from build123d import *

# Parameters (mm, degrees)
F1_DEPTH = 7.5
F2_R     = 5
F3_DEPTH = 10.001
F5_DEPTH = 10.001


with BuildPart() as f1:
    # F0 (on Front) → F1 (new body, symmetric)
    with BuildSketch(Plane.XZ):
        with BuildLine():
            Line((0, 10), (0, 0))
            Line((0, 0), (27.023239, 0))
            ThreePointArc((27.023239, 0), (29.876277, 0.415629), (32.492154, 1.627965))
            Line((32.492154, 1.627965), (44.251915, 9.309865))
            ThreePointArc((44.251915, 9.309865), (46.867792, 10.522202), (49.72083, 10.937831))
            Line((49.72083, 10.937831), (86.744069, 10.937831))
            Line((86.744069, 10.937831), (86.744069, 20.937831))
            Line((86.744069, 20.937831), (49.72083, 20.937831))
            ThreePointArc((49.72083, 20.937831), (46.867792, 20.522202), (44.251915, 19.309865))
            Line((44.251915, 19.309865), (32.492154, 11.627965))
            ThreePointArc((32.492154, 11.627965), (29.876277, 10.415629), (27.023239, 10))
            Line((27.023239, 10), (0, 10))
        make_face()
    extrude(amount=F1_DEPTH, both=True)

    # F2 (on face) → F3 (cut, through all)
    with BuildSketch(Plane.XY.offset(10)):
        with Locations((10, 0)):
            Circle(F2_R)
    extrude(amount=-F3_DEPTH, mode=Mode.SUBTRACT)

    # F4 (on face) → F5 (cut, through all)
    with BuildSketch(Plane.XY.offset(10)):
        with BuildLine():
            ThreePointArc((3.385622, -7.5), (0.885622, -4.114378), (0, 0))
            Line((0, 0), (0, -7.5))
            Line((0, -7.5), (3.385622, -7.5))
        make_face()
        with BuildLine():
            ThreePointArc((0, 0), (0.885622, 4.114378), (3.385622, 7.5))
            Line((3.385622, 7.5), (0, 7.5))
            Line((0, 7.5), (0, 0))
        make_face()
    extrude(amount=-F5_DEPTH, mode=Mode.SUBTRACT)


solid = f1.part
Part model, mm, in its own coordinate system. A direction names the side the tool comes from. Give positions to 0.01 mm unless a question says otherwise; leave off trailing zeros. Write each loop counter-clockwise with the first axis right and the second up, starting at its lowest first coordinate (ties: lowest second). Pieces come first, ordered by that corner, then holes.
1) Cut at A-A on x = 10. Write the cut outline in (y, z).
Resolved:
outline: (-7.5, 0) - (-5, 0) - (-5, 10) - (-7.5, 10) - close; (5, 0) - (7.5, 0) - (7.5, 10) - (5, 10) - close
2) Pin check, flat tips, straight feed: pin 1 (2 mm diameter, centred on y = -5.5, z = 15, fed in from -X); pin 2 (8 mm diameter, centred on x = 72, y = -2.5, fed in from -Z); pin 3 (5 mm diameter, centred on y = 4, z = 7, fed in from -X); pin 4 (6 mm diameter, centred on x = 10, y = 0, fed in from -Z). Stop position of each tip, or through.
Resolved:
pin 1: stops at x = 36.12
pin 2: stops at z = 10.94
pin 3: stops at x = 0.11
pin 4: passes through
3) Two-plate mould, pull along Z, no slides. Class faces 4 (the face through (86.744, 0, 16)), 5 (the face through (29.92, -0.11, 10.43)), 6 (the face through (46.8, -0.1, 10.5)): released by +Z, released by -Z, zero draft, split by the parting line, or undercut.
Resolved:
face 4: zero draft
face 5: released by +Z
face 6: released by -Z
4) Cut at D-D on y = 6. Write the cut outline in (x, z).
Resolved:
outline: (2, 0) - (27.02, 0) arc R10 ccw to (32.49, 1.63) - (44.25, 9.31) arc R10 cw to (49.72, 10.94) - (86.74, 10.94) - (86.74, 20.94) - (49.72, 20.94) arc R10 ccw to (44.25, 19.31) - (32.49, 11.63) arc R10 cw to (27.02, 10) - (2, 10) - close
5) Probe L1, parallel to Y at x = 10, z = 4.75; L2, parallel to Z at x = 50.5, y = -5.25; L3, parallel to X at y = 3, z = 4.5. List the from-to ranges inside material, lowest first.
Resolved:
L1: y = -7.5 to -5, 5 to 7.5
L2: z = 10.94 to 20.94
L3: x = 0.46 to 6, 14 to 36.89
6) Cut at B-B on y = 2.25. Write the cut outline in (x, z), then the cut area to 3 significant figures.
Resolved:
outline: (0.26, 0) - (5.53, 0) - (5.53, 10) - (0.26, 10) - close; (14.47, 0) - (27.02, 0) arc R10 ccw to (32.49, 1.63) - (44.25, 9.31) arc R10 cw to (49.72, 10.94) - (86.74, 10.94) - (86.74, 20.94) - (49.72, 20.94) arc R10 ccw to (44.25, 19.31) - (32.49, 11.63) arc R10 cw to (27.02, 10) - (14.47, 10) - close
area: 776 mm2
7) Which spindle directions (+Z, -Z, +X, -X, +Y, -Y) get a long thin tool onto all of the face, cutting with end or side? Do faces 1 (the face through (14.77, 1.5, 5.07)), 2 (the face through (68, 0, 10.938)), 3 (the face through (17, 0, 10)). Say none if no direction does.
Resolved:
face 1: +Z, -Z
face 2: -Z, +X, +Y, -Y
face 3: +Z, -X, +Y, -Y
8) Cut at C-C on z = 5. Write the cut outline in (x, y).
Resolved:
outline: (0, 0) arc R10 ccw to (3.39, -7.5) - (37.65, -7.5) - (37.65, 7.5) - (3.39, 7.5) arc R10 ccw to start; hole circle Ø10 at (10, 0)
